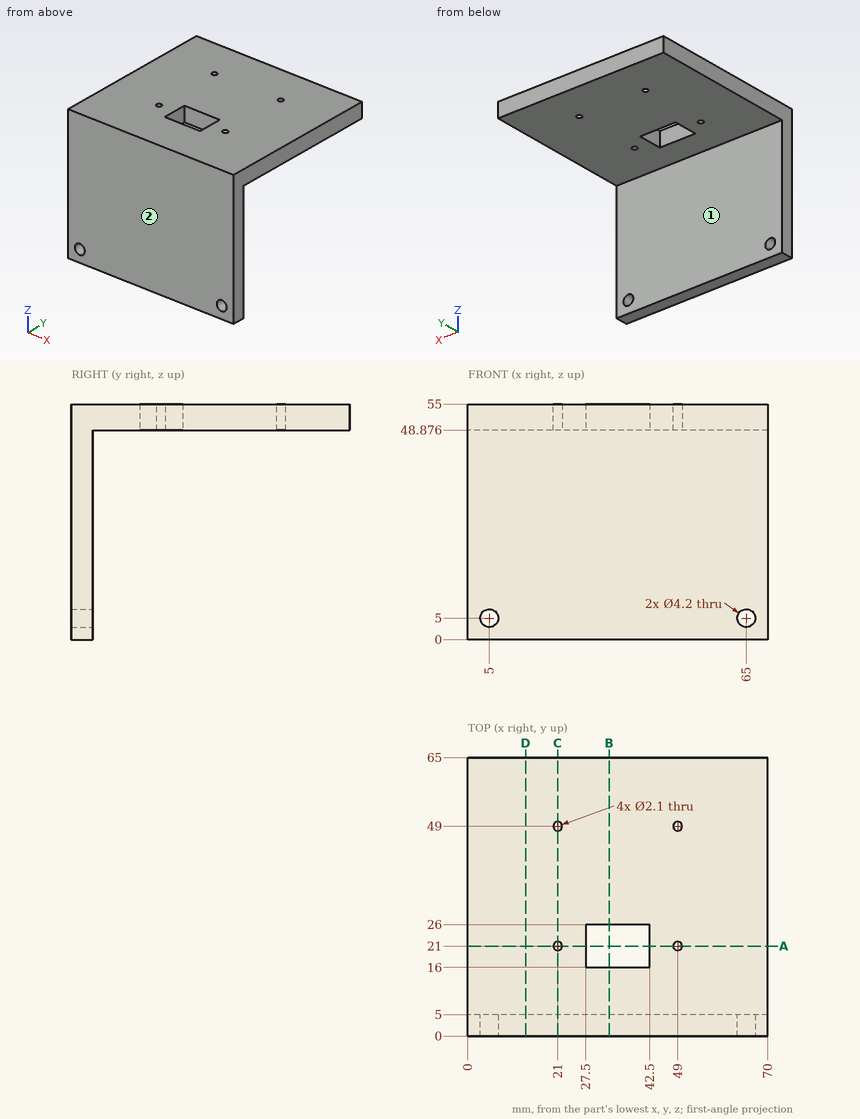
Design review of the part shown in the three views and the two pictorial views. Dimensions are in mm from the part's minimum x, y and z. A direction names the side the tool comes from. Give positions to 0.01 mm unless a question says otherwise; leave off trailing zeros. Write each loop counter-clockwise with the first axis right and the second up, starting at its lowest first coordinate (ties: lowest second). Pieces come first, ordered by that corner, then holes. Notation, with made-up numbers: (83, -16.5) - (122, -16.5) arc R22 ccw to (122, 2.5) - close; hole circle Ø3 at (68.5, 21.5). An arc over 180 degrees is marked (long way). Return JSON: item names as keys, results as strings. Group by question number.
(1) To check wall thickness, follow probe 1 along Y at (x, z) = (21, 51.75); probe 2 along Z at (x, y) = (48.5, 13); probe 3 along Y at (x, z) = (40.5, 8.5). State the ranges of each line that lie inside material, in increasing order.
(2) Insertion check: pin 1 (18 mm diameter, centred on x = 44.5, y = 27.5, fed in from -Z); pin 2 (6 mm diameter, centred on x = 54, z = 42.5, fed in from +Y). Each pin has a flat end and moves straight along its axis. Give the tip position at first contact, or say it passes through.
(3) We need section B-B, the plane x = 33. Give the boundary of the cut face in (y, z).
(4) We need section D-D, the plane x = 13.5. Give the boundary of the cut face in (y, z).
(5) Machinability: for the marked faces 1 and 2, which of the approach directions +Z, -Z, +X, -X, +Y, -Y give a long, thin tool a straight path to every point of the face, cutting with its end or side? Answer none if there is none.
(6) We need section C-C, the plane x = 21. Give the boundary of the cut face in (y, z).
(7) We need section A-A, the plane y = 21. Give the boundary of the cut face in (x, z), then the cut area to 3 significant figures.
Reported:
{
 "1": {"probe 1": "y = 0 to 19.95, 22.05 to 47.95, 50.05 to 65", "probe 2": "z = 48.88 to 55", "probe 3": "y = 0 to 5"},
 "2": {"pin 1": "stops at z = 48.88", "pin 2": "stops at y = 5"},
 "3": {"outline": "(0, 0) - (5, 0) - (5, 48.88) - (16, 48.88) - (16, 55) - (0, 55) - close; (26, 48.88) - (65, 48.88) - (65, 55) - (26, 55) - close"},
 "4": {"outline": "(0, 0) - (5, 0) - (5, 48.88) - (65, 48.88) - (65, 55) - (0, 55) - close"},
 "5": {"face 1": "-Z, +X, -X, +Y", "face 2": "+Z, -Z, +X, -X, -Y"},
 "6": {"outline": "(0, 0) - (5, 0) - (5, 48.88) - (19.95, 48.88) - (19.95, 55) - (0, 55) - close; (22.05, 48.88) - (47.95, 48.88) - (47.95, 55) - (22.05, 55) - close; (50.05, 48.88) - (65, 48.88) - (65, 55) - (50.05, 55) - close"},
 "7": {"outline": "(0, 48.88) - (19.95, 48.88) - (19.95, 55) - (0, 55) - close; (22.05, 48.88) - (27.5, 48.88) - (27.5, 55) - (22.05, 55) - close; (42.5, 48.88) - (47.95, 48.88) - (47.95, 55) - (42.5, 55) - close; (50.05, 48.88) - (70, 48.88) - (70, 55) - (50.05, 55) - close", "area": "311 mm2"}
}
